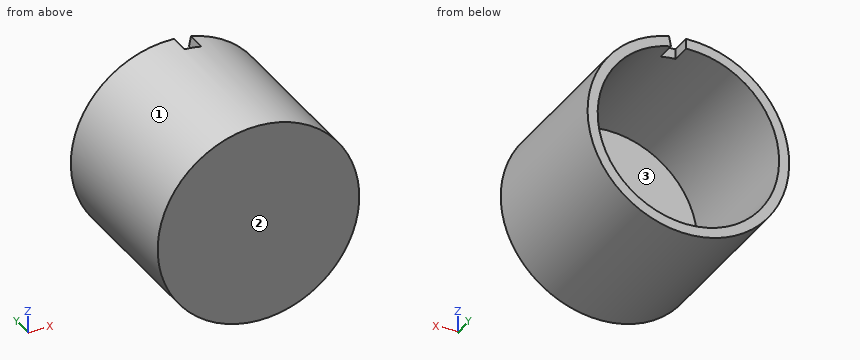
```python
from build123d import *

# Parameters (mm, degrees)
SKETCH1_R           = 15
BOSS_EXTRUDE1_DEPTH = 25
SHELL2_T            = -1.5
CUT_EXTRUDE1_START  = -3
CUT_EXTRUDE1_DEPTH  = 3


with BuildPart() as part:
    # Sketch1 → Boss-Extrude1 (new body)
    with BuildSketch(Plane(origin=(0, 0, 0), x_dir=(1, 0, 0), z_dir=(0, 1, 0))):
        with Locations(Location((0, 0, 0), (0, 0, 270))):
            Circle(SKETCH1_R)
    extrude(amount=BOSS_EXTRUDE1_DEPTH)

    # Shell2
    shell2_openings = [part.faces().sort_by_distance(p)[0] for p in [
        (0, 25, 0),
    ]]
    offset(amount=SHELL2_T, openings=shell2_openings, kind=Kind.INTERSECTION)

    # Sketch2 → Cut-Extrude1 (cut)
    with BuildSketch(Plane(origin=(0, 25, 0), x_dir=(1, 0, 0), z_dir=(0, 1, 0)).offset(CUT_EXTRUDE1_START)):
        with BuildLine():
            Line((0.356193266, -13.495300158), (0.395770296, -14.994777953))
            ThreePointArc((0.395770296, -14.994777953), (1.642962601, -14.909750967), (2.878743851, -14.721169581))
            Line((2.878743851, -14.721169581), (2.590869465, -13.249052623))
            ThreePointArc((2.590869465, -13.249052623), (1.478666341, -13.41877587), (0.356193266, -13.495300158))
        make_face()
    extrude(amount=CUT_EXTRUDE1_DEPTH, mode=Mode.SUBTRACT)


solid = part.part
```
The model under review builds one solid part; all positions refer to its coordinate system, in mm. Face numbers are marked on the shaded views. Round coordinates to 2 decimals unless told otherwise and drop trailing zeros. Loops run counter-clockwise (first coordinate to the right, second up) from the corner with the lowest first, then second, coordinate; pieces in that order, holes last. Notation, with made-up numbers: (-39, 6.25) -> (2, 6.25) arc R24 cw to (2, 43.25) -> close; hole circle Ø8 at (74.25, -0.75). An arc over 180 degrees is marked (long way). Answer in a Markdown table with one row per item.
1) Draft analysis for pull direction Z (two halves, no side actions). For the marked faces 1, 2 and 3, state which applies: pulls with the +Z half, pulls with the -Z half, needs draft (parallel to the pull), parting line crosses it, or undercut.
Taken from the geometry:
| item | result |
|---|---|
| face 1 | parting line crosses it |
| face 2 | needs draft |
| face 3 | undercut |
2) Consider section B-B, the plane x = -4.5. Write out the cut boundary in (y, z), plus the area to 3 significant figures.
Taken from the geometry:
| item | result |
|---|---|
| outline | (0, -14.31) -> (25, -14.31) -> (25, -12.73) -> (1.5, -12.73) -> (1.5, 12.73) -> (25, 12.73) -> (25, 14.31) -> (0, 14.31) -> close |
| area | 117 mm² |
3) Consider section C-C, the plane y = 17. Write out the cut boundary in (x, z).
Taken from the geometry:
| item | result |
|---|---|
| outline | circle Ø30 at (0, 0); hole circle Ø27 at (0, 0) |
4) For pin 1 Ø5 at (x, z) = (-5.5, -7.5) entering from +Y; pin 2 Ø8 at (x, y) = (10.5, 14) entering from -Z; pin 3 Ø6 at (x, y) = (-6, 14) entering from +Z, all flat-tipped, find the tip position at first contact; note any pin that passes through.
Taken from the geometry:
| item | result |
|---|---|
| pin 1 | stops at y = 1.5 |
| pin 2 | stops at z = -13.52 |
| pin 3 | stops at z = 14.7 |
5) Wall thickness on line 1 along X through (y, z) = (20.25, 0); line 2 along Y through (x, z) = (-0.75, 2); line 3 along X through (y, z) = (4.25, 6.75): over which ranges is each line inside the solid? List them lowest first.
Taken from the geometry:
| item | result |
|---|---|
| line 1 | x = -15 to -13.5, 13.5 to 15 |
| line 2 | y = 0 to 1.5 |
| line 3 | x = -13.4 to -11.69, 11.69 to 13.4 |
6) Consider section A-A, the plane z = 0. Write out the cut boundary in (x, y).
Taken from the geometry:
| item | result |
|---|---|
| outline | (-15, 0) -> (15, 0) -> (15, 25) -> (13.5, 25) -> (13.5, 1.5) -> (-13.5, 1.5) -> (-13.5, 25) -> (-15, 25) -> close |
